from build123d import *

# Parameters (mm, degrees)
PAD_DEPTH    = 1
PAD001_DEPTH = 0.5


with BuildPart() as part:
    # Sketch → Pad (new body)
    with BuildSketch(Plane.XY):
        with BuildLine():
            Line((2, 5.5), (2, -5.5))
            Line((2, -5.5), (-2, -5.5))
            Line((-2, -5.5), (-2, 5.5))
            ThreePointArc((2, 5.5), (0, 5.683346), (-2, 5.5))
        make_face()
    extrude(amount=PAD_DEPTH)

    # Sketch001 → Pad001 (new body)
    with BuildSketch(Plane.XY.offset(1)):
        Polygon((-1.5, 4), (1.5, 4), (1.5, 3), (-0.3, -3), (1.5, -3), (1.5, -4), (-1.5, -4), (-1.5, -3), (0.3, 3), (-1.5, 3), align=None)
    extrude(amount=PAD001_DEPTH)


solid = part.part
Verification items for the finished model (mm, model axes). A direction names the side the tool comes from. Give positions to 0.01 mm unless a question says otherwise; leave off trailing zeros. Write each loop counter-clockwise with the first axis right and the second up, starting at its lowest first coordinate (ties: lowest second). Pieces come first, ordered by that corner, then holes.
(1) Cross-section at A-A (z = 1.4). Enter the section's corners in (x, y).
(2) Cross-section at B-B (y = -3.5). Enter the section's corners in (x, z).
(3) Access from +Z, -Z, +X, -X, +Y, -Y to the whole of each face (thin tool, end or side, straight path). Record for faces 1 (the face through (2, 0.1, 0.5)), 2 (the face through (-0.6, 0, 1.2)).
(4) Material ranges on line 1 (Y direction, x = 0.15, z = 0.15); line 2 (Z direction, x = -0.6, y = 1); line 3 (X direction, y = 3.5, z = 1.05), recorded low to high.
(5) Cross-section at D-D (y = 0.5). Enter the section's corners in (x, z).
(6) Mould release check, pull along Y, two halves, no side actions. Record for faces 3 (the face through (-1, 0, 1)), 4 (the face through (0.028, 5.683, 0.493)), 5 (the face through (0.6, 0, 1.2)), 6 (the face through (-2, -0.1, 0.5)): +Y half, -Y half, draft (parallel to the pull), parting line (faces both ways), or undercut.
(7) Cross-section at C-C (x = 0.4). Enter the section's corners in (y, z), plus the area to 3 significant figures.
Worked out:
1. outline: (-1.5, -4) - (1.5, -4) - (1.5, -3) - (-0.3, -3) - (1.5, 3) - (1.5, 4) - (-1.5, 4) - (-1.5, 3) - (0.3, 3) - (-1.5, -3) - close
2. outline: (-2, 0) - (2, 0) - (2, 1) - (1.5, 1) - (1.5, 1.5) - (-1.5, 1.5) - (-1.5, 1) - (-2, 1) - close
3. face 1: +Z, -Z, +X, +Y, -Y
3. face 2: +Z, -X
4. line 1: y = -5.5 to 5.68
4. line 2: z = 0 to 1
4. line 3: x = -1.5 to 1.5
5. outline: (-2, 0) - (2, 0) - (2, 1) - (0.75, 1) - (0.75, 1.5) - (-0.45, 1.5) - (-0.45, 1) - (-2, 1) - close
6. face 3: undercut
6. face 4: +Y half
6. face 5: undercut
6. face 6: draft
7. outline: (-5.5, 0) - (5.68, 0) - (5.68, 1) - (4, 1) - (4, 1.5) - (-0.67, 1.5) - (-0.67, 1) - (-3, 1) - (-3, 1.5) - (-4, 1.5) - (-4, 1) - (-5.5, 1) - close
7. area: 14.0 mm2
